Input: dimensioned drawing with shaded views. Units: mm. Origin: part minimum x, y, z. Round coordinates to 2 decimals unless told otherwise and drop trailing zeros. Order: outer loops, then holes, each group sorted by start corner. A loop starts at its lowest first (then second) coordinate and runs counter-clockwise, first axis right, second up.
Item 1: Cut plane B-B on z = 1.8. Give the number of separate pieces and of enclosed holes in the cut face, then the cut area to 3 significant figures.
Item 2: Cut plane A-A on x = 12.7. Output: boundary loops of the cut face in (y, z) (1 decimal).
Item 3: First-contact query: pin 1 (2.5 mm diameter, centred on x = 57.15, y = 57.15, fed in from -Z) (3 decimals); pin 2 (7 mm diameter, centred on x = 12.7, y = 12.7, fed in from +Z) (3 decimals); pin 3 (1 mm diameter, centred on y = 61.5, z = 1.5, fed in from +X); pin 4 (1 mm diameter, centred on x = 15.5, z = 2, fed in from +Y). Flat tips, straight axial feed; report the tip coordinate or a pass-through.
Item 4: Line query: L1, parallel to Y at x = 12.7, z = 1.6; L2, parallel to Y at x = 57.15, z = 2.45; L3, parallel to Y at x = 58, z = 2.15. Output: solid intervals per line, ascending.
Item 5: Cut plane C-C on y = 12.7. Output: boundary loops of the cut face in (x, z) (1 decimal), then the cut area to 3 significant figures.
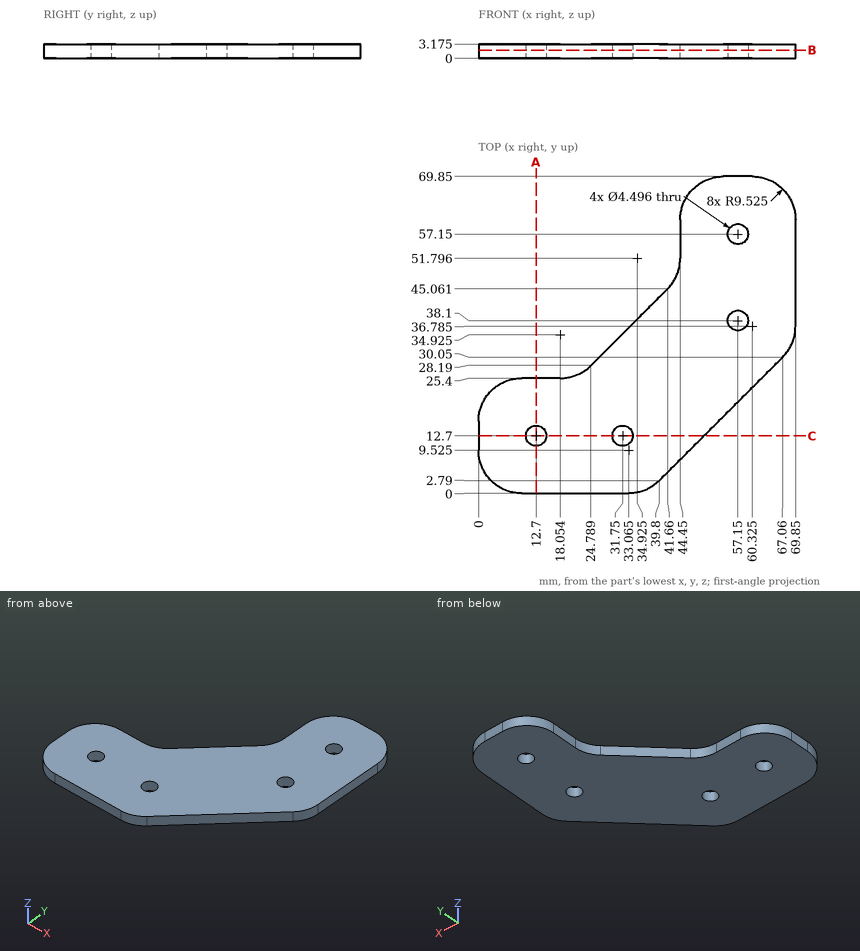
From the geometry:
1. separate pieces: 1
1. enclosed holes: 4
1. area: 2,470 mm2
2. outline: (0, 0) - (10.5, 0) - (10.5, 3.2) - (0, 3.2) - close; (14.9, 0) - (25.4, 0) - (25.4, 3.2) - (14.9, 3.2) - close
3. pin 1: passes through
3. pin 2: stops at z = 3.175
3. pin 3: stops at x = 69.83
3. pin 4: stops at y = 25.4
4. L1: y = 0 to 10.45, 14.95 to 25.4
4. L2: y = 20.14 to 35.85, 40.35 to 54.9, 59.4 to 69.85
4. L3: y = 20.99 to 36.02, 40.18 to 55.07, 59.23 to 69.85
5. outline: (0, 0) - (10.5, 0) - (10.5, 3.2) - (0, 3.2) - close; (14.9, 0) - (29.5, 0) - (29.5, 3.2) - (14.9, 3.2) - close; (34, 0) - (49.7, 0) - (49.7, 3.2) - (34, 3.2) - close
5. area: 129 mm2
